Geometry check sheet. Reference: drawing and pictorial views, mm from the part's lowest x, y, z. Give positions to 0.01 mm unless a question says otherwise; leave off trailing zeros. Loops run counter-clockwise (first coordinate to the right, second up) from the corner with the lowest first, then second, coordinate; pieces in that order, holes last. Notation, with made-up numbers: (-28, 68.5) -> (5, 68.5) arc R17 ccw to (5, 79.5) -> close; hole circle Ø9 at (10, 64.25). An arc over 180 degrees is marked (long way). Write each question's results on one line, items separated by ' | '. Start each with the question number.
1. Cross-section at A-A on x = 27. Record the boundary of the cut face in (y, z).
2. Material ranges on L1, parallel to Y at x = 43.5, z = 2.25; L2, parallel to X at y = 59, z = 2, recorded low to high. Write a range as from..to.
3. Cross-section at B-B on y = 33.5. Record the boundary of the cut face in (x, z), and give its area (3 significant figures).
4. Gauge pin test, flat ends, axial feed: pin 1 Ø3 at (x, z) = (68.5, 2.5) entering from -Y; pin 2 Ø2.5 at (y, z) = (91, 1.5) entering from -X; pin 3 Ø2.5 at (x, z) = (3, 3) entering from +Y. Record the tip position at first contact, or that the pin passes through.
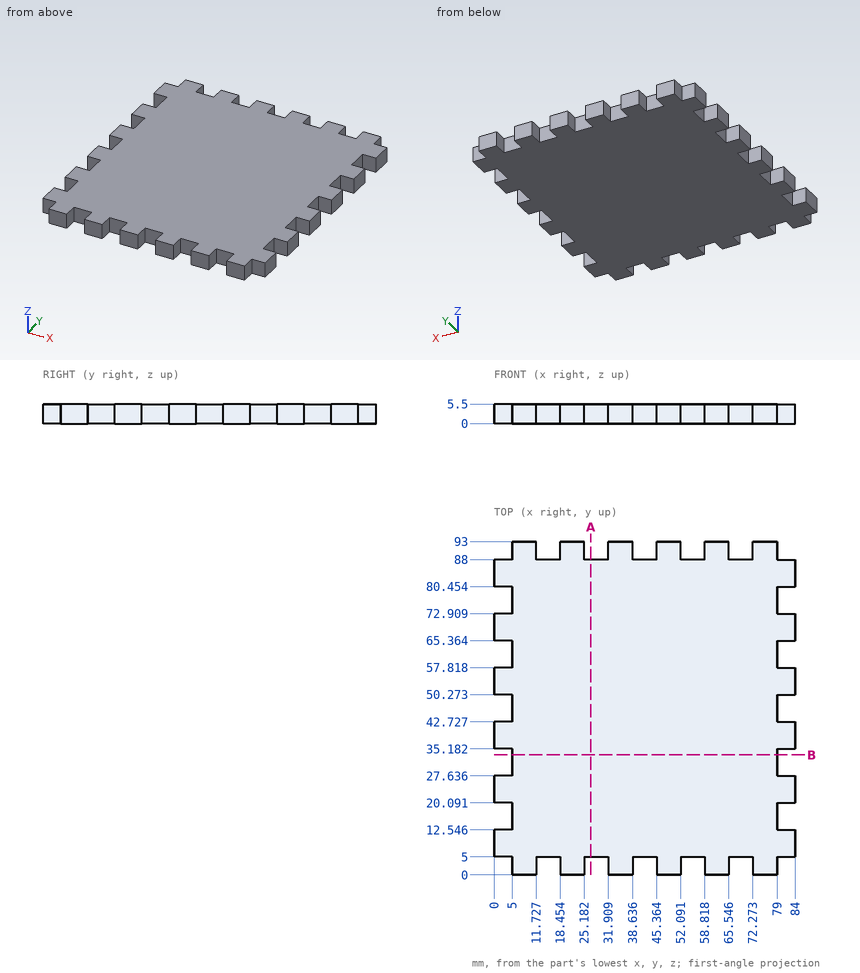
Geometry says:
1) outline: (5, 0) -> (88, 0) -> (88, 5.5) -> (5, 5.5) -> close
2) L1: 5..88 | L2: 5..79
3) outline: (5, 0) -> (79, 0) -> (79, 5.5) -> (5, 5.5) -> close | area: 407 mm^2
4) pin 1: y = 5 | pin 2: x = 5 | pin 3: y = 88
